Autodesk Inventor part; units mm, degrees
ref_plane "YZ Plane" through (0, 0, 0) normal (1, 0, 0) x (0, 1, 0)
ref_plane "XZ Plane" through (0, 0, 0) normal (0, 1, 0) x (-1, 0, 0)
ref_plane "XY Plane" through (0, 0, 0) normal (0, 0, 1) x (1, 0, 0)
sketch "Náčrt12" plane through (0, 0, 0) normal (0, 1, 0) x (-1, 0, 0)
  line L0 (0, 0) -> (177.8, 0)
  line L1 (177.8, 0) -> (177.8, 50.8)
  line L2 (177.8, 50.8) -> (0, 50.8)
  line L3 (0, 50.8) -> (0, 0)
  dimension "d34" = 50.8
  dimension "d35" = 177.8
extrude "Vysunutí10" add sketch "Náčrt12" along normal blind 2.54
sketch "Náčrt13" plane through (0, 0, 0) normal (0, -1, 0) x (1, 0, 0)
  line L0 (0, 50.8) -> (0, 0)
  line L1 (-177.8, 50.8) -> (0, 50.8)
  line L2 (-177.8, 0) -> (-177.8, 50.8)
  line L3 (0, 0) -> (-177.8, 0)
  line L4 (-175.26, 0) -> (-175.26, 48.26)
  line L5 (-175.26, 48.26) -> (-2.54, 48.26)
  line L6 (-2.54, 48.26) -> (-2.54, 0)
  line L7 (-175.26, 10.16) -> (-2.54, 10.16)
  line L8 (-2.54, 10.16) -> (-2.54, 7.62)
  line L9 (-2.54, 7.62) -> (-175.26, 7.62)
  line L10 (-175.26, 7.62) -> (-175.26, 10.16)
  line L11 (-175.26, 22.86) -> (-2.54, 22.86)
  line L12 (-2.54, 22.86) -> (-2.54, 20.32)
  line L13 (-2.54, 20.32) -> (-175.26, 20.32)
  line L14 (-175.26, 20.32) -> (-175.26, 22.86)
  line L15 (-175.26, 35.56) -> (-2.54, 35.56)
  line L16 (-2.54, 35.56) -> (-2.54, 33.02)
  line L17 (-2.54, 33.02) -> (-175.26, 33.02)
  line L18 (-175.26, 33.02) -> (-175.26, 35.56)
  line L19 (-175.26, 40.64) -> (-2.54, 40.64)
  line L20 (-2.54, 40.64) -> (-2.54, 38.1)
  line L21 (-2.54, 38.1) -> (-175.26, 38.1)
  line L22 (-175.26, 38.1) -> (-175.26, 40.64)
  line L23 (-175.26, 15.24) -> (-2.54, 15.24)
  line L24 (-2.54, 15.24) -> (-2.54, 12.7)
  line L25 (-2.54, 12.7) -> (-175.26, 12.7)
  line L26 (-175.26, 12.7) -> (-175.26, 15.24)
  line L27 (-175.26, 27.94) -> (-2.54, 27.94)
  line L28 (-2.54, 27.94) -> (-2.54, 25.4)
  line L29 (-2.54, 25.4) -> (-175.26, 25.4)
  line L30 (-175.26, 25.4) -> (-175.26, 27.94)
  dimension "d73" = 2.54
extrude "Vysunutí11" add sketch "Náčrt13" along normal blind 43.18 contours L0 L3 L6 L5 L4 L2 L1
sketch "Náčrt14" plane through (0, 0, 0) normal (0, -1, 0) x (1, 0, 0)
  line L0 (-2.54, 0) -> (-2.54, 48.26)
  line L1 (-175.26, 48.26) -> (-175.26, 0)
  line L2 (-2.54, 0) -> (-175.26, 0)
  line L3 (-175.26, 9.525) -> (-2.54, 9.525)
  line L4 (-2.54, 9.525) -> (-2.54, 11.43)
  line L5 (-2.54, 11.43) -> (-175.26, 11.43)
  line L6 (-175.26, 11.43) -> (-175.26, 9.525)
  line L7 (-175.26, 15.24) -> (-2.54, 15.24)
  line L8 (-2.54, 15.24) -> (-2.54, 13.335)
  line L9 (-2.54, 13.335) -> (-175.26, 13.335)
  line L10 (-175.26, 13.335) -> (-175.26, 15.24)
  line L11 (-175.26, 24.13) -> (-2.54, 24.13)
  line L12 (-2.54, 24.13) -> (-2.54, 22.225)
  line L13 (-2.54, 22.225) -> (-175.26, 22.225)
  line L14 (-175.26, 22.225) -> (-175.26, 24.13)
  line L15 (-175.26, 27.94) -> (-2.54, 27.94)
  line L16 (-2.54, 27.94) -> (-2.54, 26.035)
  line L17 (-2.54, 26.035) -> (-175.26, 26.035)
  line L18 (-175.26, 26.035) -> (-175.26, 27.94)
  line L19 (-175.26, 40.64) -> (-2.54, 40.64)
  line L20 (-2.54, 40.64) -> (-2.54, 38.735)
  line L21 (-2.54, 38.735) -> (-175.26, 38.735)
  line L22 (-175.26, 38.735) -> (-175.26, 40.64)
  line L23 (-175.26, 36.83) -> (-2.54, 36.83)
  line L24 (-2.54, 36.83) -> (-2.54, 34.925)
  line L25 (-2.54, 34.925) -> (-175.26, 34.925)
  line L26 (-175.26, 34.925) -> (-175.26, 36.83)
  point P0 (0, 0)
  dimension "d59" = 11.43
  dimension "d60" = 1.905
  dimension "d61" = 1.905
  dimension "d62" = 1.905
  dimension "d63" = 1.905
  dimension "d64" = 1.905
  dimension "d65" = 1.905
  dimension "d66" = 1.905
  dimension "d67" = 10.795
  dimension "d68" = 1.905
  dimension "d69" = 10.795
  dimension "d70" = 1.905
extrude "Vysunutí12" add sketch "Náčrt14" along normal blind 1.905 contours L3 L1 L5 L0 | L9 L1 L7 L0 | L13 L1 L11 L0 | L17 L1 L15 L0 | L25 L1 L23 L0 | L21 L1 L19 L0
sketch "Náčrt16" plane through (0, -1.905, 0) normal (0, -1, 0) x (1, 0, 0)
  line L0 (-2.54, 9.525) -> (-175.26, 9.525)
  line L1 (-175.26, 11.43) -> (-173.3563, 11.43)
  line L2 (-173.3563, 11.43) -> (-173.3563, 9.525)
  line L3 (-173.3563, 9.525) -> (-175.26, 9.525)
  line L4 (-175.26, 9.525) -> (-175.26, 11.43)
  line L5 (-2.54, 11.43) -> (-4.435, 11.43)
  line L6 (-4.435, 11.43) -> (-4.435, 9.525)
  line L7 (-4.435, 9.525) -> (-2.54, 9.525)
  line L8 (-2.54, 9.525) -> (-2.54, 11.43)
  point P0 (0, 0)
extrude "Vysunutí13" add sketch "Náčrt16" along normal up to surface (41.275 mm away)
sketch "Náčrt17" plane through (0, -1.905, 0) normal (0, -1, 0) x (1, 0, 0)
  line L0 (-2.54, 13.335) -> (-175.26, 13.335)
  line L1 (-175.26, 15.24) -> (-173.3476, 15.24)
  line L2 (-173.3476, 15.24) -> (-173.3476, 13.335)
  line L3 (-173.3476, 13.335) -> (-175.26, 13.335)
  line L4 (-175.26, 13.335) -> (-175.26, 15.24)
  line L5 (-2.54, 15.24) -> (-4.4371, 15.24)
  line L6 (-4.4371, 15.24) -> (-4.4371, 13.335)
  line L7 (-4.4371, 13.335) -> (-2.54, 13.335)
  line L8 (-2.54, 13.335) -> (-2.54, 15.24)
  point P0 (0, 0)
extrude "Vysunutí14" add sketch "Náčrt17" along normal up to surface (41.275 mm away)
sketch "Náčrt18" plane through (0, -1.905, 0) normal (0, -1, 0) x (1, 0, 0)
  line L0 (-175.26, 34.925) -> (-175.26, 36.83)
  line L1 (-175.26, 34.925) -> (-2.54, 34.925)
  line L2 (-175.26, 36.83) -> (-173.3455, 36.83)
  line L3 (-173.3455, 36.83) -> (-173.3455, 34.925)
  line L4 (-173.3455, 34.925) -> (-175.26, 34.925)
  line L5 (-175.26, 34.925) -> (-175.26, 36.83)
  line L6 (-2.54, 36.83) -> (-4.4393, 36.83)
  line L7 (-4.4393, 36.83) -> (-4.4393, 34.925)
  line L8 (-4.4393, 34.925) -> (-2.54, 34.925)
  line L9 (-2.54, 34.925) -> (-2.54, 36.83)
  point P0 (0, 0)
extrude "Vysunutí15" add sketch "Náčrt18" along normal up to surface (41.275 mm away)
sketch "Náčrt19" plane through (0, -1.905, 0) normal (0, -1, 0) x (1, 0, 0)
  line L0 (-175.26, 38.735) -> (-175.26, 40.64)
  line L1 (-2.54, 38.735) -> (-175.26, 38.735)
  line L2 (-175.26, 40.64) -> (-173.3529, 40.64)
  line L3 (-173.3529, 40.64) -> (-173.3529, 38.735)
  line L4 (-173.3529, 38.735) -> (-175.26, 38.735)
  line L5 (-175.26, 38.735) -> (-175.26, 40.64)
  line L6 (-2.54, 40.64) -> (-4.4393, 40.64)
  line L7 (-4.4393, 40.64) -> (-4.4393, 38.735)
  line L8 (-4.4393, 38.735) -> (-2.54, 38.735)
  line L9 (-2.54, 38.735) -> (-2.54, 40.64)
  point P0 (0, 0)
extrude "Vysunutí16" add sketch "Náčrt19" along normal up to surface (41.275 mm away)
sketch "Náčrt20" plane through (0, -43.18, 0) normal (0, -1, 0) x (1, 0, 0)
  line L0 (-175.26, 40.64) -> (-175.26, 48.26)
  line L1 (0, 50.8) -> (-177.8, 50.8)
  line L2 (-170.18, 50.8) -> (-149.86, 50.8)
  line L3 (-149.86, 50.8) -> (-149.86, 48.26)
  line L4 (-149.86, 48.26) -> (-170.18, 48.26)
  line L5 (-170.18, 48.26) -> (-170.18, 50.8)
  dimension "d83" = 20.32
  dimension "d84" = 25.4
extrude "Vysunutí17" cut sketch "Náčrt20" against normal blind 9.525
sketch "Náčrt21" plane through (0, 0, 0) normal (0, -1, 0) x (1, 0, 0)
  line L0 (-175.26, 15.24) -> (-2.54, 15.24)
  line L1 (-2.54, 13.335) -> (-175.26, 13.335)
  line L2 (-2.54, 24.13) -> (-175.26, 24.13)
  ellipse E0 centre (-127, 18.7502) end of major axis (-116.84, 18.7502) minor radius 3.175
  ellipse E1 centre (-50.8, 18.7502) end of major axis (-40.64, 18.7502) minor radius 3.175
  line L3 (-2.54, 0) -> (-175.26, 0)
  line L4 (-175.26, 22.225) -> (-175.26, 15.24)
  point P0 (0, 0)
  dimension "d92" = 10.16
  dimension "d93" = 10.16
  dimension "d122" = 3.175
  dimension "d120" = 18.7502
  dimension "d121" = 48.26
  dimension "d123" = 76.2
extrude "Vysunutí18" add sketch "Náčrt21" along normal up to surface (43.18 mm away)
sketch "Náčrt22" plane through (-127, -43.18, 18.7502) normal (0, -1, 0) x (1, 0, 0)
  ellipse E0 centre (0, 0) end of major axis (-10.16, 0) minor radius 3.175
  circle A0 centre (0, 0) radius 0.9525
  point P0 (127, -18.7502)
  dimension "d96" = 1.905
extrude "Vysunutí19" cut sketch "Náčrt22" against normal blind 20.32 contours A0
sketch "Náčrt23" plane through (-50.8, -43.18, 18.7502) normal (0, -1, 0) x (1, 0, 0)
  ellipse E0 centre (0, 0) end of major axis (-10.16, 0) minor radius 3.175
  circle A0 centre (0, 0) radius 0.9525
  point P0 (50.8, -18.7502)
  dimension "d99" = 1.905
extrude "Vysunutí20" cut sketch "Náčrt23" against normal blind 20.32 contours A0
sketch "Náčrt24" plane through (0, -43.18, 0) normal (0, -1, 0) x (1, 0, 0)
  line L0 (-149.86, 50.8) -> (-149.86, 48.26)
  line L1 (-2.54, 48.26) -> (-2.54, 40.64)
  line L2 (-2.54, 0) -> (0, 0)
  line L3 (0, 0) -> (0, 50.8)
  line L4 (0, 50.8) -> (-149.86, 50.8)
  line L5 (-1.27, 0) -> (-1.27, 49.53)
  line L6 (-1.27, 49.53) -> (-149.86, 49.53)
extrude "Vysunutí21" add sketch "Náčrt24" along normal blind 1.27
sketch "Náčrt25" plane through (0, -43.18, 0) normal (0, -1, 0) x (1, 0, 0)
  line L0 (-170.18, 48.26) -> (-170.18, 50.8)
  line L1 (-170.18, 50.8) -> (-177.8, 50.8)
  line L2 (-177.8, 50.8) -> (-177.8, 0)
  line L3 (-177.8, 0) -> (-175.26, 0)
  line L4 (-175.26, 48.26) -> (-170.18, 48.26)
  line L5 (-176.53, 0) -> (-176.53, 49.53)
  line L6 (-176.53, 49.53) -> (-170.18, 49.53)
  point P0 (0, 0)
extrude "Vysunutí22" add sketch "Náčrt25" along normal blind 1.27
sketch "Náčrt27" plane through (-2.54, 0, 27.94) normal (-1, 0, 0) x (0, 0, 1)
  circle A0 centre (-9.2075, -10.16) radius 4.445
  point P0 (-27.94, 0)
  dimension "d110" = 8.89
extrude "Vysunutí23" add sketch "Náčrt27" along normal blind 12.7
sketch "Náčrt28" plane through (-15.24, -10.16, 18.7325) normal (-1, 0, 0) x (0, 0, 1)
  circle A0 centre (0, 0) radius 4.445
  circle A1 centre (0, 0) radius 0.9525
  point P0 (-18.7325, 10.16)
  dimension "d113" = 1.905
extrude "Vysunutí24" cut sketch "Náčrt28" against normal through all contours A1
sketch "Náčrt30" plane through (-175.26, 0, 22.225) normal (1, 0, 0) x (0, 0, -1)
  circle A0 centre (3.4925, -10.16) radius 4.445
  point P0 (22.225, 0)
extrude "Vysunutí25" add sketch "Náčrt30" along normal blind 12.7
sketch "Náčrt31" plane through (-162.56, -10.16, 18.7325) normal (1, 0, 0) x (0, 0, -1)
  circle A0 centre (0, 0) radius 0.9525
  point P0 (18.7325, 10.16)
extrude "Vysunutí26" cut sketch "Náčrt31" against normal through all
properties part number "Krabicka_dolna_cast"
For this review, take the finished solid that the model builds, in its own axes (mm). A direction names the side the tool comes from. Coordinates: 2 decimals unless noted, no trailing zeros. Order: outer loops, then holes, each group sorted by start corner. A loop starts at its lowest first (then second) coordinate and runs counter-clockwise, first axis right, second up. Notation, with made-up numbers: (-27, 57.5) - (-7, 57.5) arc R26 ccw to (-7, 87.5) - close; hole circle Ø7 at (65, 23). An arc over 180 degrees is marked (long way). Answer as a JSON object with one key per item and string values. Group by question number.
1. The part is to be moulded in two halves that separate along X. For faces 5 (the flat face through (-177.8, -21, 26)), 6 (the flat face through (-75, -44.45, 50)), 7 (the flat face through (-89, -1, 36.83)), say which applies: pulls with the +X half, pulls with the -X half, needs draft (parallel to the pull), parting line crosses it, or undercut.
2. Clearance check with flat-ended pins moving along their axes: P1, Ø0.6, axis at x = -124.5, z = 10.5, coming from the -Y side (3 decimals); P2, Ø10, axis at x = -51.5, y = -10, coming from the -Z side; P3, Ø1, axis at x = -84.5, y = -12, coming from the -Z side. State where each tip first meets the part, or that it passes through.
3. We need section B-B on z = 4. State the section outline as (x, y) points.
4. For faces 1 (the flat face through (-88, 0, 31)), 2 (the flat face through (-162.56, -9, 19)), 3 (the flat face through (-88, 0, 19)), 4 (the flat face through (0, -21, 25)), list the 3-axis set-ups (+Z, -Z, +X, -X, +Y, -Y) from which the entire face can be reached by the end or side of a thin tool; tool diameter is ignored.
5. We need section C-C on y = -29. Give the number of separate pieces and of enclosed holes in the cut face, then the cut area to 3 significant figures.
6. For probe 1 along Z at (x, y) = (-50.8, -37); probe 2 along Z at (x, y) = (-10, -10); probe 3 along X at (y, z) = (-40.5, 32.5), list the stretches that pass through material, from the lowest coordinate up.
Final values:
{
 "1": {"face 5": "pulls with the -X half", "face 6": "needs draft", "face 7": "undercut"},
 "2": {"P1": "y = -1.905", "P2": "z = 15.58", "P3": "z = 48.26"},
 "3": {"outline": "(-177.8, -44.45) - (-176.53, -44.45) - (-176.53, -43.18) - (-175.26, -43.18) - (-175.26, 0) - (-2.54, 0) - (-2.54, -43.18) - (-1.27, -43.18) - (-1.27, -44.45) - (0, -44.45) - (0, 2.54) - (-177.8, 2.54) - close"},
 "4": {"face 1": "-Y", "face 2": "-Z, -Y", "face 3": "none", "face 4": "+Z, -Z, +X, +Y, -Y"},
 "5": {"separate pieces": "3", "enclosed holes": "2", "area": "923 mm²"},
 "6": {"probe 1": "15.58 to 17.8, 19.7 to 21.93, 48.26 to 50.8", "probe 2": "14.29 to 17.79, 19.67 to 23.17, 48.26 to 50.8", "probe 3": "-177.8 to -175.26, -2.54 to 0"}
}
